```python
from build123d import *

# Parameters (mm, degrees)
SKETCH2_W           = 796
SKETCH2_H           = 53
SKETCH2_R           = 5
SKETCH2_R_2         = 3.75
BOSS_EXTRUDE1_DEPTH = 20
SKETCH2_3_R         = 5
SKETCH2_3_R_2       = 3.75
CUT_EXTRUDE1_DEPTH  = 799.013157786
BOSS_EXTRUDE2_START = -8
BOSS_EXTRUDE2_DEPTH = 56
LPATTERN1_COUNT     = 4
LPATTERN1_PITCH     = 244


with BuildPart() as part:
    # Sketch2 → Boss-Extrude1 (new body)
    # profile 1 of 4: a face of its own
    with BuildSketch(Plane(origin=(0, 0, 0), x_dir=(1, 0, 0), z_dir=(0, 1, 0))):
        with Locations((398, 26.5)):
            Rectangle(SKETCH2_W, SKETCH2_H)
        with Locations((776, 15)):
            Circle(SKETCH2_R, mode=Mode.SUBTRACT)
        with Locations((776, 35)):
            Circle(SKETCH2_R_2, mode=Mode.SUBTRACT)
        with Locations((752, 15)):
            Circle(SKETCH2_R, mode=Mode.SUBTRACT)
    # profile 2 of 4: a face of its own
    with BuildSketch(Plane(origin=(0, 0, 0), x_dir=(1, 0, 0), z_dir=(0, 1, 0))):
        with Locations((752, 15)):
            Circle(SKETCH2_R)
    # profile 3 of 4: a face of its own
    with BuildSketch(Plane(origin=(0, 0, 0), x_dir=(1, 0, 0), z_dir=(0, 1, 0))):
        with Locations((776, 15)):
            Circle(SKETCH2_R)
    # profile 4 of 4: a face of its own
    with BuildSketch(Plane(origin=(0, 0, 0), x_dir=(1, 0, 0), z_dir=(0, 1, 0))):
        with Locations((776, 35)):
            Circle(SKETCH2_R_2)
    extrude(amount=BOSS_EXTRUDE1_DEPTH)

    # Sketch2_3 → Cut-Extrude1 (cut, symmetric)
    with BuildSketch(Plane(origin=(0, 0, 0), x_dir=(1, 0, 0), z_dir=(0, 1, 0))):
        with Locations(Location((752, 15, 0), (0, 0, 270))):
            Circle(SKETCH2_3_R)
        with Locations(Location((776, 15, 0), (0, 0, 270))):
            Circle(SKETCH2_3_R)
        with Locations(Location((776, 35, 0), (0, 0, 270))):
            Circle(SKETCH2_3_R_2)
    cut_extrude1 = extrude(amount=CUT_EXTRUDE1_DEPTH, both=True, mode=Mode.SUBTRACT)

    # Sketch3 → Boss-Extrude2 (add)
    with BuildSketch(Plane(origin=(796, 0, 0), x_dir=(0, 0, -1), z_dir=(1, 0, 0)).offset(BOSS_EXTRUDE2_START)):
        with BuildLine():
            Line((50.625, 20), (46.625, 20))
            Line((46.625, 20), (46.625, 26))
            Line((46.625, 26), (47.344131154, 26))
            ThreePointArc((47.344131154, 26), (48.625, 25.625), (49.905868846, 26))
            Line((49.905868846, 26), (50.625, 26))
            Line((50.625, 26), (50.625, 20))
        make_face()
    boss_extrude2 = extrude(amount=-BOSS_EXTRUDE2_DEPTH)

    # LPattern1: Cut-Extrude1, Boss-Extrude2 ×4
    with Locations(*[(-i * LPATTERN1_PITCH, 0, 0) for i in range(1, LPATTERN1_COUNT)]):
        add(cut_extrude1, mode=Mode.SUBTRACT)
        add(boss_extrude2)


solid = part.part
```
Part model, mm, in its own coordinate system. Coordinates: 2 decimals unless noted, no trailing zeros. Write each loop counter-clockwise with the first axis right and the second up, starting at its lowest first coordinate (ties: lowest second). Pieces come first, ordered by that corner, then holes.
Item 1: Slice it at B-B (x = 171). Write the cut outline in (y, z), and give its area (3 significant figures).
Item 2: Slice it at A-A (y = 15). Count the separate pieces of the cut face and the enclosed holes in it, and give its area (3 significant figures).
Item 3: Pin check, flat tips, straight feed: pin 1 (2 mm diameter, centred on x = 86, z = -25, fed in from -Y); pin 2 (10 mm diameter, centred on x = 557, z = -31, fed in from +Y); pin 3 (5 mm diameter, centred on x = 519.5, y = 23, fed in from -Z) (3 decimals); pin 4 (5 mm diameter, centred on x = 746, y = 24, fed in from +Z) (3 decimals). Stop position of each tip, or through.
Item 4: Probe line 1 (Z direction, x = 532, y = 12.5); line 2 (X direction, y = 13.75, z = -35); line 3 (Z direction, x = 752, y = 10.75). List the from-to ranges inside material, lowest first.
Results found:
1. outline: (0, -53) - (20, -53) - (20, 0) - (0, 0) - close
1. area: 1,060 mm2
2. separate pieces: 1
2. enclosed holes: 12
2. area: 41,400 mm2
3. pin 1: stops at y = 0
3. pin 2: stops at y = 20
3. pin 3: stops at z = -50.625
3. pin 4: stops at z = -46.625
4. line 1: z = -53 to -38.75, -31.25 to -20, -10 to 0
4. line 2: x = 0 to 40.25, 47.75 to 284.25, 291.75 to 528.25, 535.75 to 772.25, 779.75 to 796
4. line 3: z = -53 to -20, -10 to 0
